For this review, take the finished solid that the model builds, in its own axes (mm). Face numbers are marked on the shaded views. A direction names the side the tool comes from. Give positions to 0.01 mm unless a question says otherwise; leave off trailing zeros. Write each loop counter-clockwise with the first axis right and the second up, starting at its lowest first coordinate (ties: lowest second). Pieces come first, ordered by that corner, then holes. Notation, with made-up numbers: (53.5, -39) -> (58.5, -39) arc R21 cw to (58.5, -24) -> close; hole circle Ø5 at (-14, 89). An arc over 180 degrees is marked (long way). Write item = value, one per line.
```python
from build123d import *

# Parameters (mm, degrees)
F0_W     = 31.75
F0_H     = 31.75
F1_DEPTH = 92.075
F0_R     = 15.875
F2_DEPTH = 53.975
F3_DEPTH = 34.925
F0_H_2   = 88.9
F4_DEPTH = 73.025
F5_DEPTH = 31.75


with BuildPart() as f1:
    # F0 (on Top) → F1 (new body)
    with BuildSketch(Plane.XY):
        with Locations((-45.519012, 57.172301)):
            Rectangle(F0_W, F0_H)
        with Locations((-45.519012, -63.477699)):
            Rectangle(F0_W, F0_H)
        with Locations((62.430988, 57.172301)):
            Rectangle(F0_W, F0_H)
        with Locations((62.430988, -63.477699)):
            Rectangle(F0_W, F0_H)
    extrude(amount=F1_DEPTH)

    # F0 (on Top) → F2 (join)
    with BuildSketch(Plane.XY):
        Polygon((-29.644012, -47.602699), (-29.644012, -79.352699), (46.555988, -79.352699), (46.555988, -47.602699), (46.555988, 41.297301), (46.555988, 73.047301), (-29.644012, 73.047301), (-29.644012, 41.297301), align=None)
        with Locations((8.455988, -3.152699)):
            Circle(F0_R, mode=Mode.SUBTRACT)
    extrude(amount=F2_DEPTH)

    # F0 (on Top) → F3 (join)
    with BuildSketch(Plane.XY):
        with Locations((8.455988, -3.152699)):
            Circle(F0_R)
    extrude(amount=F3_DEPTH)



with BuildPart() as f4:
    # F0 (on Top) → F4 (new body)
    with BuildSketch(Plane.XY):
        with Locations((-45.519012, -3.152699)):
            Rectangle(F0_W, F0_H_2)
        with Locations((62.430988, -3.152699)):
            Rectangle(F0_W, F0_H_2)
    extrude(amount=F4_DEPTH)


with BuildPart() as f1_1:
    add(f1.part)

    add(f4.part)  # F5 merges F4
    # F0 (on Top) → F5 (join)
    with BuildSketch(Plane.XY):
        Polygon((-118.544012, -28.552699), (-118.544012, -79.352699), (-61.394012, -79.352699), (-61.394012, -47.602699), (-61.394012, 41.297301), (-61.394012, 73.047301), (-118.544012, 73.047301), (-118.544012, 22.247301), (-77.269012, 22.247301), (-77.269012, -28.552699), align=None)
        Polygon((78.305988, -47.602699), (78.305988, -79.352699), (135.455988, -79.352699), (135.455988, -28.552699), (94.180988, -28.552699), (94.180988, 22.247301), (135.455988, 22.247301), (135.455988, 73.047301), (78.305988, 73.047301), (78.305988, 41.297301), align=None)
    extrude(amount=F5_DEPTH)


solid = f1_1.part
```
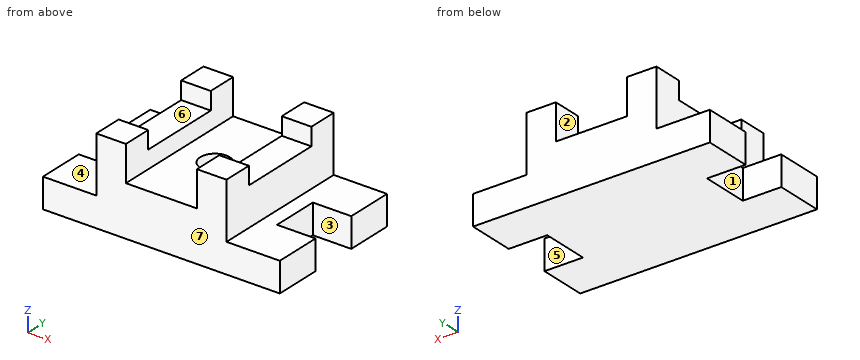
(1) For pin 1 (18 mm diameter, centred on y = -30, z = 58.5, fed in from +X); pin 2 (16 mm diameter, centred on y = -4, z = 23.5, fed in from +X); pin 3 (19 mm diameter, centred on y = -28, z = 81.5, fed in from -X), all flat-tipped, find the tip position at first contact; note any pin that passes through.
Answers below:
pin_1 = 78.31
pin_2 = 94.18
pin_3 = -61.39
(2) Take a section at B-B (x = 105.5). Write out the cut boundary in (y, z).
Answers below:
outline = (-79.35, 0) -> (-28.55, 0) -> (-28.55, 31.75) -> (-79.35, 31.75) -> close; (22.25, 0) -> (73.05, 0) -> (73.05, 31.75) -> (22.25, 31.75) -> close
(3) Tool access review of the marked faces 1, 2 and 3: name each direction out of +Z, -Z, +X, -X, +Y, -Y from which nothing blocks a thin tool from reaching the whole face with its end or side.
Answers below:
face_1 = +Z, -Z, -X
face_2 = +Z, +Y, -Y
face_3 = +Z, -Z, +X
(4) The part is to be moulded in two halves that separate along Y. For the marked faces 4, 5, 6 and 7, say which applies: released by +Y, released by -Y, zero draft, split by the parting line, or undercut.
Answers below:
face_4 = zero draft
face_5 = undercut
face_6 = undercut
face_7 = released by -Y
(5) Take a section at C-C (y = -35). Write out the cut boundary in (x, z) (3 decimals), plus the area to 3 significant figures.
Answers below:
outline = (-118.544, 0) -> (135.456, 0) -> (135.456, 31.75) -> (78.306, 31.75) -> (78.306, 73.025) -> (46.556, 73.025) -> (46.556, 53.975) -> (-29.644, 53.975) -> (-29.644, 73.025) -> (-61.394, 73.025) -> (-61.394, 31.75) -> (-118.544, 31.75) -> close
area = 12,400 mm^2
(6) Take a section at D-D (x = 72.5). Write out the cut boundary in (y, z) (3 decimals), plus the area to 3 significant figures.
Answers below:
outline = (-79.353, 0) -> (73.047, 0) -> (73.047, 92.075) -> (41.297, 92.075) -> (41.297, 73.025) -> (-47.603, 73.025) -> (-47.603, 92.075) -> (-79.353, 92.075) -> close
area = 12,300 mm^2
(7) To check wall thickness, follow probe 1 along X at (y, z) = (45.5, 68.5); probe 2 along Z at (x, y) = (85.5, 0); probe 3 along Z at (x, y) = (26, 60) (3 decimals). State the ranges of each line that lie inside material, in increasing order.
Answers below:
probe_1 = -61.39 to -29.64, 46.56 to 78.31
probe_2 = 0 to 31.75
probe_3 = 0 to 53.975
(8) Take a section at A-A (z = 59). Write out the cut boundary in (x, y).
Answers below:
outline = (-61.39, -79.35) -> (-29.64, -79.35) -> (-29.64, 73.05) -> (-61.39, 73.05) -> close; (46.56, -79.35) -> (78.31, -79.35) -> (78.31, 73.05) -> (46.56, 73.05) -> close
